Design review of the part built by this model. Coordinates are the model's own, in mm. Give positions to 0.01 mm unless a question says otherwise; leave off trailing zeros. Write each loop counter-clockwise with the first axis right and the second up, starting at its lowest first coordinate (ties: lowest second). Pieces come first, ordered by that corner, then holes. Notation, with made-up numbers: (9, 55) -> (63, 55) arc R5 cw to (63, 64) -> close; hole circle Ø11 at (21.25, 7). An arc over 180 degrees is marked (long way). Use CSV: the item, a comma, the result in double quotes.
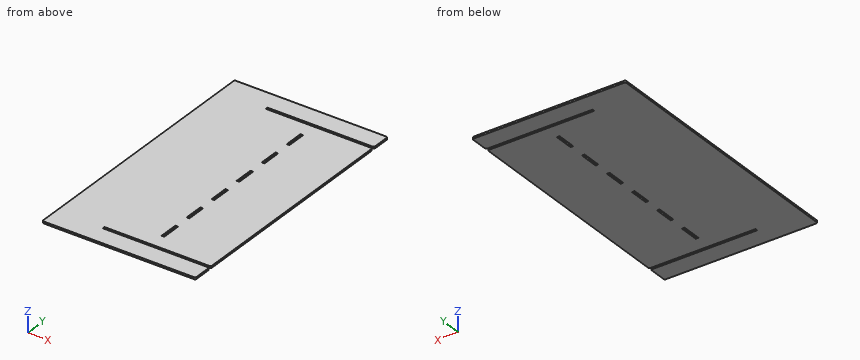
```python
from build123d import *

# Parameters (mm, degrees)
F0_W     = 397
F0_H     = 700
F1_DEPTH = 5
F2_W     = 276
F2_H     = 6
F3_DEPTH = 25
F4_W     = 7
F4_H     = 50
F5_DEPTH = 25
F6_R     = 4


with BuildPart() as f1:
    # F0 (on Top) → F1 (new body)
    with BuildSketch(Plane.XY):
        Rectangle(F0_W, F0_H)
    extrude(amount=F1_DEPTH)

    # F2 (on face) → F3 (cut)
    with BuildSketch(Plane.XY.offset(5)):
        with Locations((60.5, -297)):
            Rectangle(F2_W, F2_H)
        with Locations((60.5, 297)):
            Rectangle(F2_W, F2_H)
    extrude(amount=-F3_DEPTH, mode=Mode.SUBTRACT)

    # F4 (on face) → F5 (cut)
    with BuildSketch(Plane.XY.offset(5)):
        with Locations((45, 45.5714285714)):
            Rectangle(F4_W, F4_H)
        with Locations((45, 136.7142857143)):
            Rectangle(F4_W, F4_H)
        with Locations((45, 227.8571428571)):
            Rectangle(F4_W, F4_H)
        with Locations((45, -45.5714285714)):
            Rectangle(F4_W, F4_H)
        with Locations((45, -136.7142857143)):
            Rectangle(F4_W, F4_H)
        with Locations((45, -227.8571428571)):
            Rectangle(F4_W, F4_H)
    extrude(amount=-F5_DEPTH, mode=Mode.SUBTRACT)

    # F6
    f6_edges = [f1.edges().sort_by_distance(p)[0] for p in [
        (-198.5, -350, 2.5),
        (198.5, -350, 2.5),
        (198.5, -300, 2.5),
        (198.5, -294, 2.5),
        (198.5, 294, 2.5),
        (198.5, 300, 2.5),
        (198.5, 350, 2.5),
        (-198.5, 350, 2.5),
    ]]
    fillet(f6_edges, radius=F6_R)


solid = f1.part
```
(1) Take a section at A-A (y = -46.5). Write out the cut boundary in (x, z), then the cut area to 3 significant figures.
Established:
outline,"(-198.5, 0) -> (41.5, 0) -> (41.5, 5) -> (-198.5, 5) -> close; (48.5, 0) -> (198.5, 0) -> (198.5, 5) -> (48.5, 5) -> close"
area,"1,950 mm2"
(2) Clearance check with a flat-ended pin moving along its axis: pin 1 (2 mm diameter, centred on x = -154.5, y = 35.5, fed in from -Z). State where the tip first meets the part, or that it passes through.
Established:
pin 1,"stops at z = 0"
(3) Take a section at C-C (z = 2.1). State how many separate pieces and enclosed holes the cut face has, then the cut area to 3 significant figures.
Established:
separate pieces,"1"
enclosed holes,"6"
area,"272,000 mm2"
(4) For line 1 along Y through (x, z) = (138.5, 4.6); line 2 along X through (y, z) = (32, 1.55); line 3 along X through (y, z) = (-296, 2.5), list the stretches that pass through material, from the lowest coordinate up. Write a range as [from, to].
Established:
line 1,"y = [-350, -300], [-294, 294], [300, 350]"
line 2,"x = [-198.5, 41.5], [48.5, 198.5]"
line 3,"x = [-198.5, -77.5]"
(5) Take a section at B-B (x = -30.5). Write out the cut boundary in (y, z), then the cut area to 3 significant figures.
Established:
outline,"(-350, 0) -> (-300, 0) -> (-300, 5) -> (-350, 5) -> close; (-294, 0) -> (294, 0) -> (294, 5) -> (-294, 5) -> close; (300, 0) -> (350, 0) -> (350, 5) -> (300, 5) -> close"
area,"3,440 mm2"
